Build history of the part. All positions in model axes, mm. A direction names the side the tool comes from. Coordinates: 2 decimals unless noted, no trailing zeros. Order: outer loops, then holes, each group sorted by start corner. A loop starts at its lowest first (then second) coordinate and runs counter-clockwise, first axis right, second up. Notation, with made-up numbers: (-6, 0) - (34, 0) arc R28 ccw to (34, 30) - close; hole circle Ø11 at (-19.5, 62). An arc over 180 degrees is marked (long way). Return JSON: item names as keys, results as strings.
from build123d import *

# Parameters (mm, degrees)
BOSS_EXTRUDE1_DEPTH = 3.5
SKETCH2_R           = 1.5
BOSS_EXTRUDE2_DEPTH = 8.5
SKETCH3_R           = 1
BOSS_EXTRUDE3_DEPTH = 5


with BuildPart() as part:
    # Sketch1 → Boss-Extrude1 (new body)
    with BuildSketch(Plane.XY):
        with BuildLine():
            Line((-44.435656646, 8.394675461), (0.564343354, 8.394675461))
            ThreePointArc((0.564343354, 8.394675461), (2.314343354, 10.144675461), (0.564343354, 11.894675461))
            Line((0.564343354, 11.894675461), (-44.435656646, 11.894675461))
            ThreePointArc((-44.435656646, 11.894675461), (-46.185656646, 10.144675461), (-44.435656646, 8.394675461))
        make_face()
    extrude(amount=BOSS_EXTRUDE1_DEPTH)

    # Sketch2 → Boss-Extrude2 (add)
    with BuildSketch(Plane.XY.offset(3.5)):
        with Locations((-44.435656646, 10.144675461)):
            Circle(SKETCH2_R)
    extrude(amount=BOSS_EXTRUDE2_DEPTH)

    # Sketch3 → Boss-Extrude3 (add)
    with BuildSketch(Plane.XY.offset(3.5)):
        with Locations((0.564343354, 10.144675461)):
            Circle(SKETCH3_R)
    extrude(amount=BOSS_EXTRUDE3_DEPTH)


solid = part.part
1. Cut at B-B on z = 5.5. Give the cut face in (x, y), plus the area to 3 significant figures.
Check values:
{"outline": "circle Ø3 at (-44.44, 10.14); circle Ø2 at (0.56, 10.14)", "area": "10.2 mm²"}
2. Cut at C-C on x = -18.5. Give the cut face in (y, z), plus the area to 4 significant figures.
Check values:
{"outline": "(8.39, 0) - (11.89, 0) - (11.89, 3.5) - (8.39, 3.5) - close", "area": "12.25 mm²"}
3. Tool access for faces 5 (the cylindrical face through (2.314, 10.106, 1.726)), 6 (the cylindrical face through (-45.5, 11.2, 7.7)), 7 (the flat face through (1, 10, 8.5)): list every direction of +Z, -Z, +X, -X, +Y, -Y with a clear straight run to the whole face (end or side of a thin tool).
Check values:
{"face 5": "+Z, -Z, +X", "face 6": "+Z", "face 7": "+Z, +X, +Y, -Y"}
4. Cut at A-A on y = 9.65. Give the cut face in (x, z), plus the area to 3 significant figures.
Check values:
{"outline": "(-46.11, 0) - (2.24, 0) - (2.24, 3.5) - (1.43, 3.5) - (1.43, 8.5) - (-0.3, 8.5) - (-0.3, 3.5) - (-43.02, 3.5) - (-43.02, 12) - (-45.85, 12) - (-45.85, 3.5) - (-46.11, 3.5) - close", "area": "202 mm²"}
5. Drop a flat-ended pin along its axis: pin 1 (1 mm diameter, centred on x = 1, y = 10.5, fed in from +Z). Give the stop position or say it passes through.
Check values:
{"pin 1": "z = 8.5"}
6. Cut at D-D on z = 1.25. Give the cut face in (x, y), plus the area to 3 significant figures.
Check values:
{"outline": "(-44.44, 8.39) - (0.56, 8.39) arc R1.75 ccw to (0.56, 11.89) - (-44.44, 11.89) arc R1.75 ccw to start", "area": "167 mm²"}
7. Mould opens along X. For faces 1 (the cylindrical face through (0.348, 9.168, 5.965)), 2 (the flat face through (-22, 10, 3.5)), 3 (the flat face through (-22, 11.895, 2)), 4 (the cylindrical face through (-46.185, 10.183, 1.726)) say: pulls with the +X half, pulls with the -X half, needs draft (parallel to the pull), parting line crosses it, or undercut.
Check values:
{"face 1": "undercut", "face 2": "undercut", "face 3": "needs draft", "face 4": "pulls with the -X half"}
8. Probe L1, parallel to X at y = 10.15, z = 8; L2, parallel to Z at x = -30, y = 10.5; L3, parallel to X at y = 9.8, z = 7. List the from-to ranges inside material, lowest first.
Check values:
{"L1": "-45.94 to -42.94, -0.44 to 1.56", "L2": "0 to 3.5", "L3": "-45.9 to -42.98, -0.37 to 1.5"}
